Can you work these out from the drawing? Everything is in mm from the part's minimum corner. Give positions to 0.01 mm unless a question says otherwise; leave off trailing zeros. Loops run counter-clockwise (first coordinate to the right, second up) from the corner with the lowest first, then second, coordinate; pieces in that order, holes last. Notation, with made-up numbers: (3, 6.25) - (49, 6.25) arc R21 cw to (49, 21.25) - close; hole circle Ø2 at (59.25, -31). An arc over 180 degrees is marked (long way). Answer in a Markdown table with one row per item.
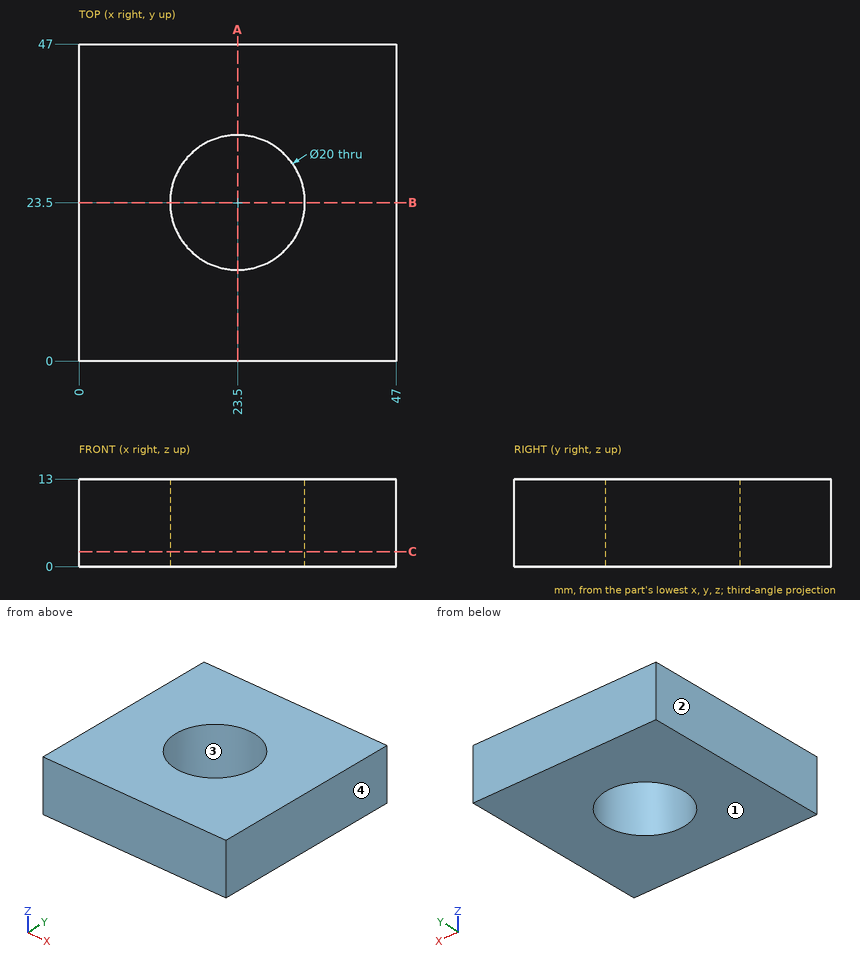
Q1. If we mould it in two halves opening along X, with no side actions, what happens to the marked faces 1, 2, 3 and 4? For each: released by +X, released by -X, zero draft, split by the parting line, or undercut.
Checked values:
| item | result |
|---|---|
| face 1 | zero draft |
| face 2 | released by -X |
| face 3 | undercut |
| face 4 | released by +X |
Q2. Imagine slicing it at A-A, the plane x = 23.5. Write out the boundary of the cut face in (y, z), and give its area (3 significant figures).
Checked values:
| item | result |
|---|---|
| outline | (0, 0) - (13.5, 0) - (13.5, 13) - (0, 13) - close; (33.5, 0) - (47, 0) - (47, 13) - (33.5, 13) - close |
| area | 351 mm² |
Q3. Imagine slicing it at C-C, the plane z = 2.25. Write out the boundary of the cut face in (x, y).
Checked values:
| item | result |
|---|---|
| outline | (0, 0) - (47, 0) - (47, 47) - (0, 47) - close; hole circle Ø20 at (23.5, 23.5) |
Q4. For pin 1 (16 mm diameter, centred on x = 23.5, y = 23.5, fed in from +Z), with a flat end and sliding along its axis, tell me the tip position at first contact or that it passes through.
Checked values:
| item | result |
|---|---|
| pin 1 | passes through |
Q5. If I drill on line 1 (Y direction, x = 23.5, z = 4); line 2 (Y direction, x = 27, z = 4); line 3 (X direction, y = 32, z = 4.75), over which ranges is the centre line in solid material (lowest first)? Write a range as [from, to].
Checked values:
| item | result |
|---|---|
| line 1 | y = [0, 13.5], [33.5, 47] |
| line 2 | y = [0, 14.13], [32.87, 47] |
| line 3 | x = [0, 18.23], [28.77, 47] |
